Autodesk Inventor part; units mm, degrees
ref_plane "YZ Plane" through (0, 0, 0) normal (1, 0, 0) x (0, 1, 0)
ref_plane "XZ Plane" through (0, 0, 0) normal (0, 1, 0) x (-1, 0, 0)
ref_plane "XY Plane" through (0, 0, 0) normal (0, 0, 1) x (1, 0, 0)
sketch "Skizze1" plane through (0, 0, 0) normal (0, 0, 1) x (1, 0, 0)
  line L0 (-40, -35) -> (40, -35)
  line L1 (40, -35) -> (40, 35)
  line L2 (40, 35) -> (-40, 35)
  line L3 (-40, 35) -> (-40, -35)
  line L4 (-40, -35) -> (40, 35) construction
  line L5 (40, -35) -> (-40, 35) construction
  point P0 (0, 0)
  dimension "d0" = 80
  dimension "d1" = 70
extrude "Extrusion1" add sketch "Skizze1" along normal blind 10
sketch "Skizze2" plane through (0, 0, 10) normal (0, 0, 1) x (1, 0, 0)
  line L0 (-40, 35) -> (-30, 35)
  line L1 (-30, 35) -> (-30, 10)
  line L2 (-30, 10) -> (-40, 10)
  line L3 (-40, 10) -> (-40, 35)
  line L4 (-40, 35) -> (-40, -35)
  line L5 (-30, -35) -> (-40, -35)
  line L6 (-40, -35) -> (-40, -10)
  line L7 (-40, -10) -> (-30, -10)
  line L8 (-30, -10) -> (-30, -35)
  line L9 (40, 35) -> (-40, 35)
  line L10 (40, -35) -> (40, 35)
  line L11 (30, 35) -> (40, 35)
  line L12 (40, 35) -> (40, 10)
  line L13 (40, 10) -> (30, 10)
  line L14 (30, 10) -> (30, 35)
  line L15 (30, -10) -> (40, -10)
  line L16 (40, -10) -> (40, -35)
  line L17 (40, -35) -> (30, -35)
  line L18 (30, -35) -> (30, -10)
  point P0 (0, 0)
  dimension "d4" = 10
  dimension "d5" = 10
  dimension "d6" = 20
  dimension "d7" = 20
  dimension "d8" = 25
  dimension "d9" = 25
extrude "Extrusion2" cut sketch "Skizze2" against normal blind 10
sketch "Skizze3" plane through (0, 0, 10) normal (0, 0, 1) x (1, 0, 0)
  line L0 (-30, -35) -> (30, -35)
  line L1 (-30, 10) -> (-40, 10)
  line L2 (40, -10) -> (40, 10)
  line L3 (30, -35) -> (30, -10)
  point P0 (0, 0)
  point P1 (24, 25)
  point P2 (24, -25)
  dimension "d12" = 10
  dimension "d13" = 50
  dimension "d17" = 16
hole "Bohrung1" at (24, 25, 10) at (24, -25, 10) direction (0, 0, -1) diameter 10 end through all
sketch "Skizze4" plane through (0, 0, 10) normal (0, 0, 1) x (1, 0, 0)
  line L0 (40, -10) -> (40, 10)
  line L1 (-30, 10) -> (-40, 10)
  point P0 (0, 0)
  point P1 (-18, 0)
  dimension "d25" = 58
  dimension "d26" = 10
hole "Bohrung2" at (-18, 0, 10) direction (0, 0, -1) diameter 15 end through all
sketch "Skizze5" plane through (-40, -10, 10) normal (0, -1, 0) x (1, 0, 0)
  line L0 (0, 0) -> (10, 0)
  line L1 (10, 0) -> (10, -10)
  point P0 (40, -10)
  point P1 (5, -5)
  dimension "d34" = 5
  dimension "d35" = 5
hole "Bohrung3" at (-35, -10, 5) direction (0, 1, 0) diameter 4 end through all
sketch "Skizze6" plane through (40, -10, 0) normal (1, 0, 0) x (0, 0, -1)
  line L0 (0, 20) -> (-10, 20)
  line L1 (0, 0) -> (0, 20)
  point P0 (0, 10)
  point P1 (-5, 10)
  dimension "d43" = 10
  dimension "d44" = 5
hole "Bohrung4" at (40, 0, 5) direction (-1, 0, 0) diameter 4 depth 10 tip angle 118
fillet "Rundung1" radius 5 2 edges at (-40, 0, 0) (-40, 0, 10)
properties part number "ABI_Deckel"
Part model, mm, in its own coordinate system. A direction names the side the tool comes from. Round coordinates to 2 decimals unless told otherwise and drop trailing zeros. Loops run counter-clockwise (first coordinate to the right, second up) from the corner with the lowest first, then second, coordinate; pieces in that order, holes last.
1. Slice it at A-A (y = -4.5). Count the separate pieces of the cut face and the enclosed holes in it, and give its area (3 significant figures).
Solutions:
separate pieces: 2
enclosed holes: 1
area: 657 mm2
2. Slice it at B-B (x = -18). Give the cut face in (y, z).
Solutions:
outline: (-35, 0) - (-7.5, 0) - (-7.5, 10) - (-35, 10) - close; (7.5, 0) - (35, 0) - (35, 10) - (7.5, 10) - close
3. Drill centre lines: line 1 along Y through (x, z) = (24, 7); line 2 along X through (y, z) = (0, 4.75); line 3 along Z through (x, y) = (36.5, 0). Where is each one in solid material? Low to high.
Solutions:
line 1: y = -35 to -30, -20 to 20, 30 to 35
line 2: x = -39.99 to -36.98, -33.02 to -25.5, -10.5 to 28.95
line 3: z = 0 to 3, 7 to 10
4. Slice it at C-C (y = 25). Give the cut face in (x, z).
Solutions:
outline: (-30, 0) - (19, 0) - (19, 10) - (-30, 10) - close; (29, 0) - (30, 0) - (30, 10) - (29, 10) - close
5. Two-plate mould, pull along Y, no slides. Class faces 6 (the face through (0, -35, 5)), 7 (the face through (34.9, 1.2, 6.6)), 8 (the face through (-25.436, 0.976, 4.93)), 9 (the face through (30, 22, 5)): pulls with the +Y half, pulls with the -Y half, needs draft (parallel to the pull), parting line crosses it, or undercut.
Solutions:
face 6: pulls with the -Y half
face 7: undercut
face 8: undercut
face 9: needs draft
6. 3-axis set-ups, long thin cutter, end or side, ignore diameter. For faces 1 (the face through (35, 10, 5)), 2 (the face through (35, -10, 5)), 3 (the face through (40, -0.1, 2.7)), 4 (the face through (-32.8, -10, 5.1)), 5 (the face through (-30, 23, 5)): which of +Z, -Z, +X, -X, +Y, -Y reach the whole face in a straight line?
Solutions:
face 1: +Z, -Z, +X, +Y
face 2: +Z, -Z, +X, -Y
face 3: +Z, -Z, +X, +Y, -Y
face 4: +Z, -Z, -X, -Y
face 5: +Z, -Z, -X, +Y
7. Flat gauge pins, fed straight in: pin 1 (1 mm diameter, centred on y = 13.5, z = 3.5, fed in from +X); pin 2 (5 mm diameter, centred on y = -28, z = 5, fed in from -X); pin 3 (5 mm diameter, centred on x = 36, z = 3.5, fed in from +Y). Where does each tip first touch, or does it go through?
Solutions:
pin 1: stops at x = 30
pin 2: stops at x = -30
pin 3: stops at y = 10
8. Slice it at D-D (x = 24). Give the cut face in (y, z), and give its area (3 significant figures).
Solutions:
outline: (-35, 0) - (-30, 0) - (-30, 10) - (-35, 10) - close; (-20, 0) - (20, 0) - (20, 10) - (-20, 10) - close; (30, 0) - (35, 0) - (35, 10) - (30, 10) - close
area: 500 mm2
